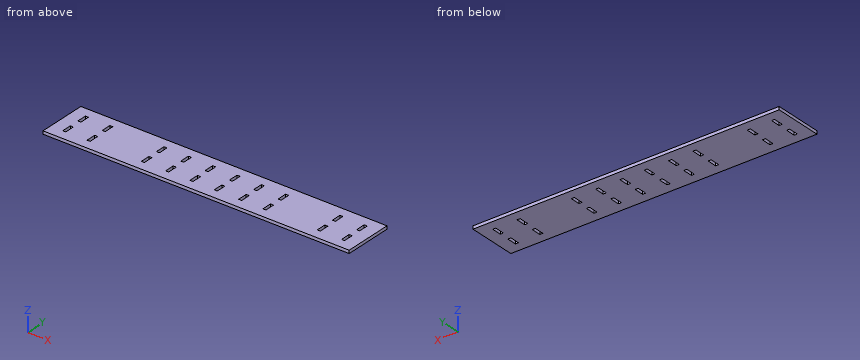
from build123d import *

# Parameters (mm, degrees)
F0_W     = 3.175
F0_H     = 10.16
F1_DEPTH = 3.175


with BuildPart() as f1:
    # F0 (on Top) → F1 (new body)
    with BuildSketch(Plane.XY):
        Polygon((-129.159, -28.17584), (190.5, -28.17584), (190.5, 22.624161), (177.8, 22.624161), (174.625, 22.624161), (152.4, 22.624161), (149.225, 22.624161), (-129.159, 22.624161), align=None)
        with Locations((-114.8715, -12.93584)):
            Rectangle(F0_W, F0_H, mode=Mode.SUBTRACT)
        with Locations((-89.4715, -12.93584)):
            Rectangle(F0_W, F0_H, mode=Mode.SUBTRACT)
        with Locations((-32.8295, -12.93584)):
            Rectangle(F0_W, F0_H, mode=Mode.SUBTRACT)
        with Locations((-7.4295, -12.93584)):
            Rectangle(F0_W, F0_H, mode=Mode.SUBTRACT)
        with Locations((17.9705, -12.93584)):
            Rectangle(F0_W, F0_H, mode=Mode.SUBTRACT)
        with Locations((43.3705, -12.93584)):
            Rectangle(F0_W, F0_H, mode=Mode.SUBTRACT)
        with Locations((68.7705, -12.93584)):
            Rectangle(F0_W, F0_H, mode=Mode.SUBTRACT)
        with Locations((94.1705, -12.93584)):
            Rectangle(F0_W, F0_H, mode=Mode.SUBTRACT)
        with Locations((150.8125, -12.93584)):
            Rectangle(F0_W, F0_H, mode=Mode.SUBTRACT)
        with Locations((176.2125, -12.93584)):
            Rectangle(F0_W, F0_H, mode=Mode.SUBTRACT)
        with Locations((-114.8715, 7.384161)):
            Rectangle(F0_W, F0_H, mode=Mode.SUBTRACT)
        with Locations((-89.4715, 7.384161)):
            Rectangle(F0_W, F0_H, mode=Mode.SUBTRACT)
        with Locations((-32.8295, 7.384161)):
            Rectangle(F0_W, F0_H, mode=Mode.SUBTRACT)
        with Locations((-7.4295, 7.384161)):
            Rectangle(F0_W, F0_H, mode=Mode.SUBTRACT)
        with Locations((17.9705, 7.384161)):
            Rectangle(F0_W, F0_H, mode=Mode.SUBTRACT)
        with Locations((43.3705, 7.384161)):
            Rectangle(F0_W, F0_H, mode=Mode.SUBTRACT)
        with Locations((68.7705, 7.384161)):
            Rectangle(F0_W, F0_H, mode=Mode.SUBTRACT)
        with Locations((94.1705, 7.384161)):
            Rectangle(F0_W, F0_H, mode=Mode.SUBTRACT)
        with Locations((150.8125, 7.384161)):
            Rectangle(F0_W, F0_H, mode=Mode.SUBTRACT)
        with Locations((176.2125, 7.384161)):
            Rectangle(F0_W, F0_H, mode=Mode.SUBTRACT)
    extrude(amount=F1_DEPTH)


solid = f1.part
The listing builds one solid part. Answer for the finished solid, in the listing's coordinates (mm). Round coordinates to 2 decimals unless told otherwise and drop trailing zeros. Use a Markdown table: item, result. Add a question column.
1. The part is cut by section A-A (y = 6). Give the number of separate pieces and of enclosed holes in the cut face, and give its area (3 significant figures).
2. Consider line 1 (Y direction, x = 43.5, z = 0.6). Determine where the line is inside the solid, lowest interval first.
3. A flat-ended cylindrical pin translates along its axis: P1, Ø5, axis at x = 43, y = 2, coming from the -Z side. Find the tip coordinate at first contact, or state that the pin passes through.
Reported:
| question | item | result |
|---|---|---|
| 1 | separate pieces | 11 |
| 1 | enclosed holes | 0 |
| 1 | area | 914 mm^2 |
| 2 | line 1 | -28.18 to -18.02, -7.86 to 2.3, 12.46 to 22.62 |
| 3 | P1 | z = 0 |
